Drawing for the job (mm, zero at the part's lowest x, y, z). Coordinates: 2 decimals unless noted, no trailing zeros. Order: outer loops, then holes, each group sorted by start corner. A loop starts at its lowest first (then second) coordinate and runs counter-clockwise, first axis right, second up. Notation, with made-up numbers: M -4.5,50.25 L 1.5,50.25 A12 ccw 1.5,60.25 Z; hole C 19,33 d2. An arc over 180 degrees is marked long. Write item = value, one per line. Start each with the question number.
Q1. Band-saw the part on A-A on y = 12. Write the cut outline in (x, z).
Q2. Band-saw the part on B-B on y = 39.5. Write the cut outline in (x, z) (1 decimal).
Q3. Drill centre lines: probe 1 along Z at (x, y) = (5, 10); probe 2 along Z at (x, y) = (19.5, 13.5); probe 3 along X at (y, z) = (9.5, 2.5). Where is each one in solid material? Low to high.
Q4. Pin check, flat tips, straight feed: P1, Ø5, axis at x = 9, y = 32, coming from the +Z side (1 decimal); P2, Ø5, axis at y = 5.5, z = 4.5, coming from the +X side; P3, Ø3, axis at y = 9, z = 11.5, coming from the -X side. Stop position of each tip, or through.
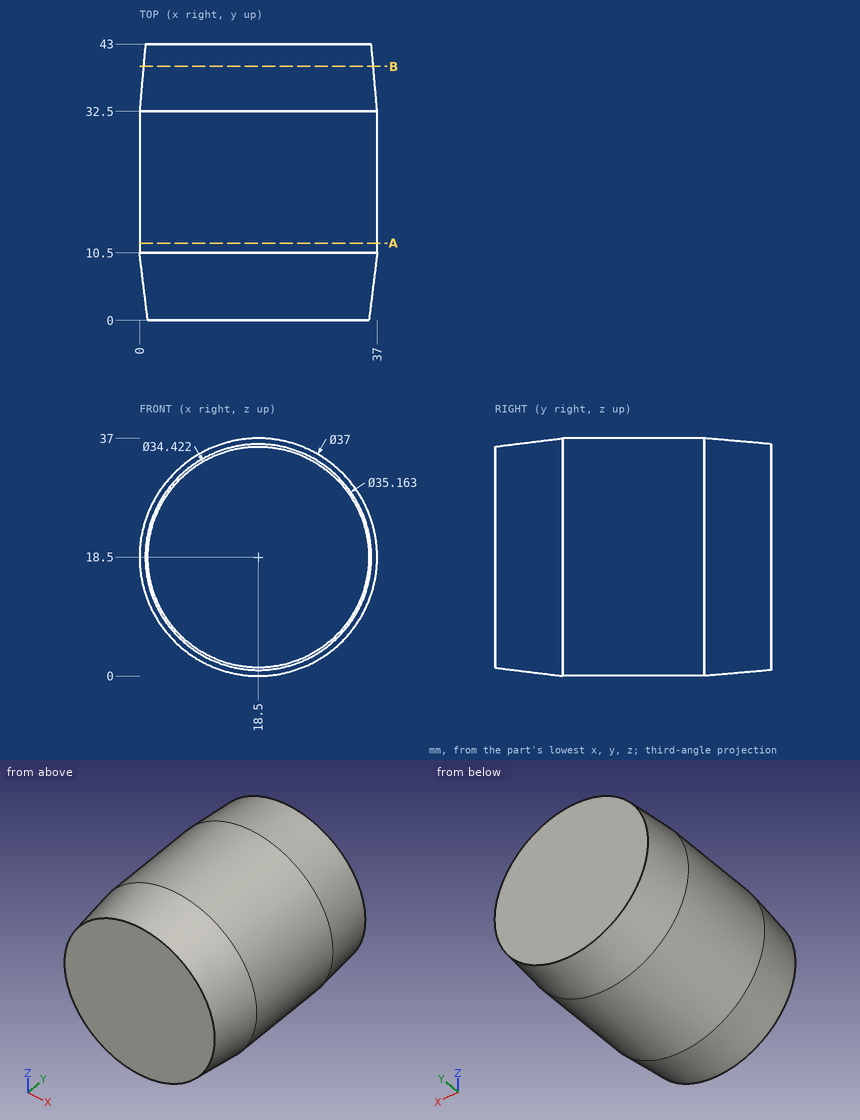
Recorded:
q1.outline = C 18.5,18.5 d37
q2.outline = C 18.5,18.5 d35.8
q3.probe_1 = 5.94 to 31.06
q3.probe_2 = 0.03 to 36.97
q3.probe_3 = 9.46 to 27.54
q4.P1 = 35.6
q4.P2 = 32.24
q4.P3 = 0.99
